The listing builds one solid part. Answer for the finished solid, in the listing's coordinates (mm). A direction names the side the tool comes from. Round coordinates to 2 decimals unless told otherwise and drop trailing zeros. Write each loop counter-clockwise with the first axis right and the second up, starting at its lowest first coordinate (ties: lowest second). Pieces come first, ordered by that corner, then holes.
(1) Find the intervals of material crossed by probe 1 along X at (y, z) = (9.75, 0); probe 2 along Z at (x, y) = (0, 11.7), in increasing order.
(2) For faces 1 (the face through (-5, 2.9, -3)), 2 (the face through (2.5, 0.345, 1.917)), 3 (the face through (-1.4, 0, -2.1)), determine the directions among +Z, -Z, +X, -X, +Y, -Y from which every point of the face is accessible in a straight line to the end or side of a thin tool.
(3) A cutting plane is placed at C-C, the plane z = -5.25. Give the vertices of the cut face in (x, y).
(4) A cutting plane is placed at D-D, the plane x = -4.75. Give the vertices of the cut face in (y, z).
(5) A cutting plane is placed at B-B, the plane y = 5.5. Give the vertices of the cut face in (x, z).
(6) Each of these flat-tipped pins is pushed along its axis until it touches: pin 1 Ø5.5 at (x, z) = (0, 0) entering from +Y; pin 2 Ø1 at (x, y) = (4, 5) entering from -Z; pin 3 Ø4 at (x, z) = (0, 0) entering from +Y; pin 4 Ø1.5 at (x, y) = (0, 8.5) entering from +Z. Where does it stop, or does it pass through?
Autodesk Inventor part; units mm, degrees
ref_plane "YZ Plane" through (0, 0, 0) normal (1, 0, 0) x (0, 1, 0)
ref_plane "XZ Plane" through (0, 0, 0) normal (0, 1, 0) x (-1, 0, 0)
ref_plane "XY Plane" through (0, 0, 0) normal (0, 0, 1) x (1, 0, 0)
sketch "Sketch1" plane through (0, 0, 0) normal (0, 1, 0) x (-1, 0, 0)
  circle A0 centre (0, 0) radius 3.15
  circle A1 centre (0, 0) radius 2.2
  dimension "d0" = 6.3
  dimension "d1" = 4.4
extrude "Extrusion1" add sketch "Sketch1" along normal blind 0.7
sketch "Sketch2" plane through (0, 0.7, 0) normal (0, 1, 0) x (1, 0, 0)
  circle A0 centre (0, 0) radius 2.2
  circle A1 centre (0, 0) radius 3.15
  circle A2 centre (0, 0) radius 6.35
  dimension "d4" = 12.7
extrude "Extrusion2" add sketch "Sketch2" along normal blind 2.2 contours A1 | A2
sketch "Sketch3" plane through (0, 2.9, 0) normal (0, 1, 0) x (1, 0, 0)
  circle A0 centre (0, 0) radius 2.2
  circle A1 centre (0, 0) radius 6.35
  circle A2 centre (0, 0) radius 5.5
  dimension "d7" = 11
extrude "Extrusion3" add sketch "Sketch3" along normal blind 8.6 contours A2
sketch "Sketch4" plane through (0, 11.5, 0) normal (0, 1, 0) x (1, 0, 0)
  circle A0 centre (0, 0) radius 2.2
  circle A1 centre (0, 0) radius 3.15
extrude "Extrusion4" add sketch "Sketch4" along normal blind 0.7
properties part number "lager" material "Stainless Steel"
Solutions:
1. probe 1: x = -5.5 to -2.2, 2.2 to 5.5
1. probe 2: z = -3.15 to -2.2, 2.2 to 3.15
2. face 1: +Y
2. face 2: -Y
2. face 3: +Z, -Z, +X, -X, -Y
3. outline: (-3.57, 0.7) - (3.57, 0.7) - (3.57, 2.9) - (1.64, 2.9) - (1.64, 11.5) - (-1.64, 11.5) - (-1.64, 2.9) - (-3.57, 2.9) - close
4. outline: (0.7, -4.21) - (2.9, -4.21) - (2.9, -2.77) - (11.5, -2.77) - (11.5, 2.77) - (2.9, 2.77) - (2.9, 4.21) - (0.7, 4.21) - close
5. outline: circle Ø11 at (0, 0); hole circle Ø4.4 at (0, 0)
6. pin 1: stops at y = 12.2
6. pin 2: stops at z = -4.24
6. pin 3: passes through
6. pin 4: stops at z = 5.5
